Geometry check sheet. Reference: the model listing, model coordinates, mm. Face numbers are marked on the shaded views. A direction names the side the tool comes from. Give positions to 0.01 mm unless a question says otherwise; leave off trailing zeros. Order: outer loops, then holes, each group sorted by start corner. A loop starts at its lowest first (then second) coordinate and runs counter-clockwise, first axis right, second up. Notation, with made-up numbers: M -38.75,80 L 15.25,80 A15 ccw 15.25,84 Z; hole C 9,52.25 d2. An arc over 180 degrees is marked long. Answer as a JSON object with one key per item and string values. Group by question number.
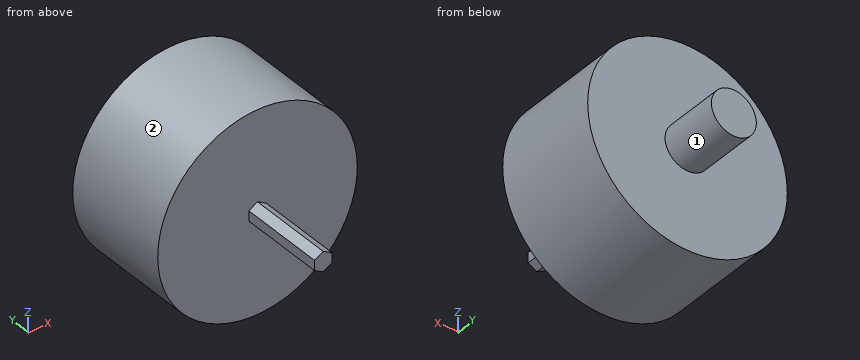
from build123d import *

# Parameters (mm, degrees)
BOSS_EXTRUDE1_DEPTH = 8.5
SKETCH2_R           = 10
BOSS_EXTRUDE2_DEPTH = 11
SKETCH3_R           = 2.25
BOSS_EXTRUDE3_DEPTH = 6


with BuildPart() as part:
    # Sketch1 → Boss-Extrude1 (new body)
    with BuildSketch(Plane(origin=(0, 0, 0), x_dir=(1, 0, 0), z_dir=(0, 1, 0))):
        Polygon((0, 1), (-0.866025404, 0.5), (-0.866025404, -0.5), (0, -1), (0.866025404, -0.5), (0.866025404, 0.5), align=None)
    extrude(amount=BOSS_EXTRUDE1_DEPTH)

    # Sketch2 → Boss-Extrude2 (add)
    with BuildSketch(Plane(origin=(0, 8.5, 0), x_dir=(1, 0, 0), z_dir=(0, 1, 0))):
        Circle(SKETCH2_R)
    extrude(amount=BOSS_EXTRUDE2_DEPTH)

    # Sketch3 → Boss-Extrude3 (add)
    with BuildSketch(Plane(origin=(0, 19.5, 0), x_dir=(1, 0, 0), z_dir=(0, 1, 0))):
        Circle(SKETCH3_R)
    extrude(amount=BOSS_EXTRUDE3_DEPTH)


solid = part.part
1. Cross-section at C-C (x = -3). Record the cut outline in (y, z), and give its area (3 significant figures).
2. Access from +Z, -Z, +X, -X, +Y, -Y to the whole of each face (thin tool, end or side, straight path). Record for the marked faces 1 and 2.
3. Thickness scan on line 1 along Y through (x, z) = (4.5, 4); line 2 along X through (y, z) = (13.5, 5); line 3 along Z through (x, y) = (-0.25, 18.5). Record the ranges inside material, lowest first. Write a range as [from, to].
4. Cross-section at D-D (y = 12.5). Record the cut outline in (x, z), and give its area (3 significant figures).
5. Cross-section at A-A (z = 0). Record the cut outline in (x, y), and give its area (3 significant figures).
6. Depth check by flat-ended pin: pin 1 (6 mm diameter, centred on x = -6, y = 21, fed in from +Z); pin 2 (8 mm diameter, centred on x = 6, z = -2.5, fed in from -Y); pin 3 (10 mm diameter, centred on x = 7.5, y = 19.5, fed in from -Z). Enter the tip coordinate at first touch or a pass-through.
7. Cross-section at B-B (y = 20). Record the cut outline in (x, z).
Report:
{
 "1": {"outline": "M 8.5,-9.54 L 19.5,-9.54 L 19.5,9.54 L 8.5,9.54 Z", "area": "210 mm2"},
 "2": {"face 1": "+Y", "face 2": "+Y, -Y"},
 "3": {"line 1": "y = [8.5, 19.5]", "line 2": "x = [-8.66, 8.66]", "line 3": "z = [-10, 10]"},
 "4": {"outline": "C 0,0 d20", "area": "314 mm2"},
 "5": {"outline": "M -10,8.5 L -0.87,8.5 L -0.87,0 L 0.87,0 L 0.87,8.5 L 10,8.5 L 10,19.5 L 2.25,19.5 L 2.25,25.5 L -2.25,25.5 L -2.25,19.5 L -10,19.5 Z", "area": "262 mm2"},
 "6": {"pin 1": "stops at z = 9.4", "pin 2": "stops at y = 8.5", "pin 3": "stops at z = -9.68"},
 "7": {"outline": "C 0,0 d4.5"}
}
